Input: dimensioned drawing with shaded views. Units: mm. Origin: part minimum x, y, z. A direction names the side the tool comes from. Round coordinates to 2 decimals unless told otherwise and drop trailing zeros. Loops run counter-clockwise (first coordinate to the right, second up) from the corner with the lowest first, then second, coordinate; pieces in that order, holes last. Notation, with made-up numbers: (78, 4) - (107, 4) arc R15 cw to (107, 21) - close; hole circle Ø4 at (-36, -15.75). An arc over 180 degrees is marked (long way). Write each question's results on one line, items separated by ' | '.
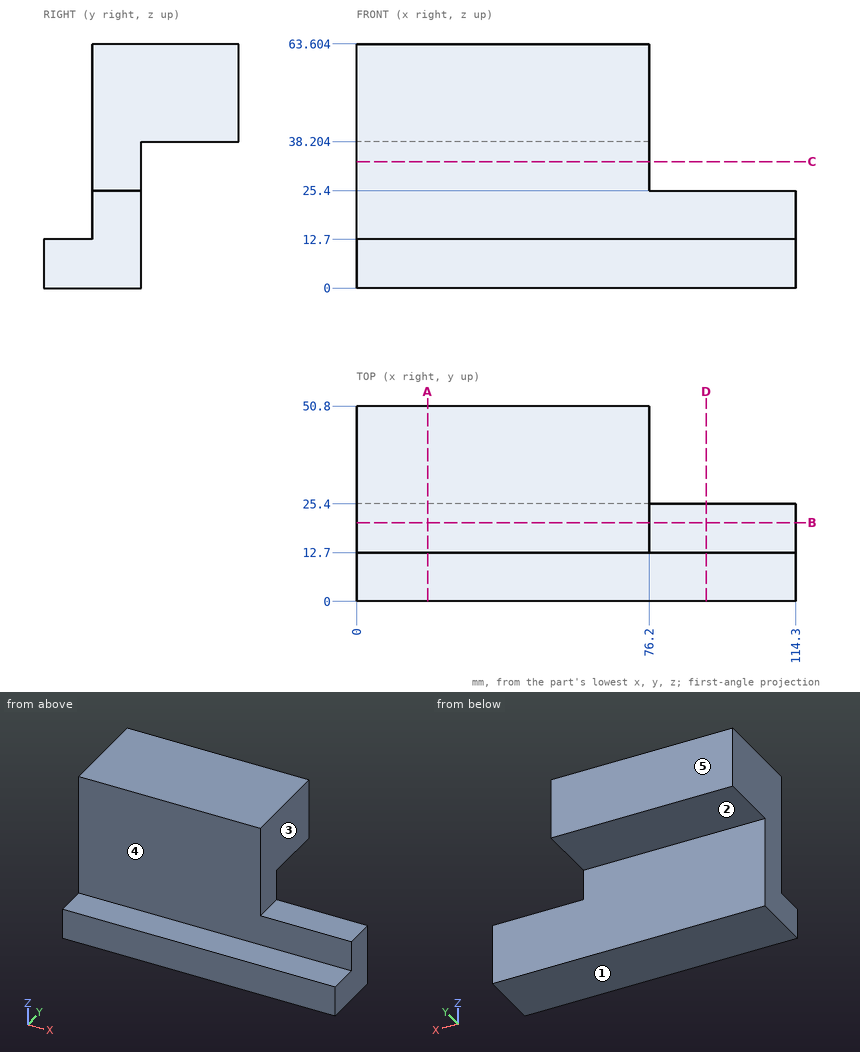
1. Section query D-D, the plane x = 91. Output: boundary loops of the cut face in (y, z).
Answer:
outline: (0, 0) - (25.4, 0) - (25.4, 25.4) - (12.7, 25.4) - (12.7, 12.7) - (0, 12.7) - close
2. Section query C-C, the plane z = 33. Output: boundary loops of the cut face in (x, y).
Answer:
outline: (0, 12.7) - (76.2, 12.7) - (76.2, 25.4) - (0, 25.4) - close
3. Section query A-A, the plane x = 18.5. Output: boundary loops of the cut face in (y, z), plus the area to 3 significant figures.
Answer:
outline: (0, 0) - (25.4, 0) - (25.4, 38.2) - (50.8, 38.2) - (50.8, 63.6) - (12.7, 63.6) - (12.7, 12.7) - (0, 12.7) - close | area: 1,610 mm^2
4. Set-up query: the marked faces 1, 2, 3, 4 and 5. Return all of +Z, -Z, +X, -X, +Y, -Y with unobstructed straight access to the full face (end or side cutting, diameter ignored); none if empty.
Answer:
face 1: -Z, +X, -X, +Y, -Y | face 2: -Z, +X, -X, +Y | face 3: +Z, +X, +Y, -Y | face 4: +Z, +X, -X, -Y | face 5: +Z, -Z, +X, -X, +Y
5. Section query B-B, the plane y = 20.5. Output: boundary loops of the cut face in (x, z), plus the area to 3 significant figures.
Answer:
outline: (0, 0) - (114.3, 0) - (114.3, 25.4) - (76.2, 25.4) - (76.2, 63.6) - (0, 63.6) - close | area: 5,810 mm^2
6. Line query: line 1 (Y direction, x = 38, z = 41.5); line 2 (Y direction, x = 74.5, z = 31.5); line 3 (X direction, y = 29, z = 57). Output: solid intervals per line, ascending. Write a range as [from, to].
Answer:
line 1: [12.7, 50.8] | line 2: [12.7, 25.4] | line 3: [0, 76.2]
7. Contact query for flat-ended pins moving along their axis: pin 1 (12 mm diameter, centred on x = 84.5, z = 12.5, fed in from +Y); pin 2 (12 mm diameter, centred on x = 65, y = 43, fed in from -Z); pin 3 (10 mm diameter, centred on x = 90, y = 19, fed in from +Z). Output: stop coordinate, or through.
Answer:
pin 1: y = 25.4 | pin 2: z = 38.2 | pin 3: z = 25.4
